The listing builds one solid part. Answer for the finished solid, in the listing's coordinates (mm). Coordinates: 2 decimals unless noted, no trailing zeros. Order: outer loops, then holes, each group sorted by start corner. A loop starts at its lowest first (then second) coordinate and runs counter-clockwise, first axis right, second up. Notation, with made-up numbers: (26.25, -34) -> (39.25, -34) arc R12 cw to (39.25, -12) -> close; hole circle Ø11 at (12.5, 35.25). An arc over 180 degrees is marked (long way). Return JSON: item names as keys, results as strings.
```python
from build123d import *

# Parameters (mm, degrees)
BOSS_EXTRUDE1_DEPTH = 1.25
BOSS_EXTRUDE5_DEPTH = 2.5
SKETCH6_W           = 5
SKETCH6_H           = 4
CUT_EXTRUDE1_DEPTH  = 1.25
CUT_EXTRUDE2_DEPTH  = 2.5


with BuildPart() as part:
    # Sketch2 → Boss-Extrude1 (new body, symmetric)
    with BuildSketch(Plane(origin=(0, 0, 0), x_dir=(1, 0, 0), z_dir=(0, 1, 0))):
        with BuildLine():
            Line((-16.109808132, 35.188266684), (-8.537351427, 63.449059844))
            ThreePointArc((-8.537351427, 63.449059844), (0, 70), (8.537351427, 63.449059844))
            Line((8.537351427, 63.449059844), (16.109808132, 35.188266684))
            ThreePointArc((16.109808132, 35.188266684), (18.609958913, 31.446526618), (22.871288916, 30))
            Line((22.871288916, 30), (37.5, 30))
            ThreePointArc((37.5, 30), (48.106601718, 25.606601718), (52.5, 15))
            Line((52.5, 15), (52.5, -15))
            ThreePointArc((52.5, -15), (40.784271247, -43.284271247), (12.5, -55))
            Line((12.5, -55), (-12.5, -55))
            ThreePointArc((-12.5, -55), (-40.784271247, -43.284271247), (-52.5, -15))
            Line((-52.5, -15), (-52.5, 15))
            ThreePointArc((-52.5, 15), (-48.106601718, 25.606601718), (-37.5, 30))
            Line((-37.5, 30), (-22.871288916, 30))
            ThreePointArc((-22.871288916, 30), (-18.609958913, 31.446526618), (-16.109808132, 35.188266684))
        make_face()
        with BuildLine():
            Line((6.122536861, 62.802012231), (13.694993566, 34.541219072))
            ThreePointArc((13.694993566, 34.541219072), (17.08805534, 29.463143267), (22.871288916, 27.5))
            Line((22.871288916, 27.5), (37.5, 27.5))
            ThreePointArc((37.5, 27.5), (46.338834765, 23.838834765), (50, 15))
            Line((50, 15), (50, -15))
            ThreePointArc((50, -15), (39.016504294, -41.516504294), (12.5, -52.5))
            Line((12.5, -52.5), (-12.5, -52.5))
            ThreePointArc((-12.5, -52.5), (-39.016504294, -41.516504294), (-50, -15))
            Line((-50, -15), (-50, 15))
            ThreePointArc((-50, 15), (-46.338834765, 23.838834765), (-37.5, 27.5))
            Line((-37.5, 27.5), (-22.871288916, 27.5))
            ThreePointArc((-22.871288916, 27.5), (-17.08805534, 29.463143267), (-13.694993566, 34.541219072))
            Line((-13.694993566, 34.541219072), (-6.122536861, 62.802012231))
            ThreePointArc((-6.122536861, 62.802012231), (0, 67.5), (6.122536861, 62.802012231))
        make_face(mode=Mode.SUBTRACT)
    extrude(amount=BOSS_EXTRUDE1_DEPTH, both=True)

    # Sketch5 → Boss-Extrude5 (add)
    with BuildSketch(Plane(origin=(0, 1.25, 0), x_dir=(1, 0, 0), z_dir=(0, 1, 0))):
        with BuildLine():
            ThreePointArc((-50, 15), (-41.161165235, 18.661165235), (-37.5, 27.5))
            ThreePointArc((-37.5, 27.5), (-46.338834765, 23.838834765), (-50, 15))
        make_face()
        with BuildLine():
            ThreePointArc((37.5, 27.5), (41.161165235, 18.661165235), (50, 15))
            ThreePointArc((50, 15), (46.338834765, 23.838834765), (37.5, 27.5))
        make_face()
        with BuildLine():
            ThreePointArc((-50, -15), (-42.291585286, -22.095919329), (-45.973512014, -31.904851181))
            ThreePointArc((-45.973512014, -31.904851181), (-48.979492188, -23.688880811), (-50, -15))
        make_face()
        with BuildLine():
            ThreePointArc((50, -15), (42.291585286, -22.095919329), (45.973512014, -31.904851181))
            ThreePointArc((45.973512014, -31.904851181), (48.979492187, -23.688880811), (50, -15))
        make_face()
    extrude(amount=-BOSS_EXTRUDE5_DEPTH)

    # Sketch6 → Cut-Extrude1 (cut)
    with BuildSketch(Plane(origin=(0, 1.25, 0), x_dir=(1, 0, 0), z_dir=(0, 1, 0))):
        with Locations((0, 68.75)):
            Rectangle(SKETCH6_W, SKETCH6_H)
        with BuildLine():
            Line((-20.493193447, 30.416333701), (-19.643873637, 28.065024308))
            ThreePointArc((-19.643873637, 28.065024308), (-17.08805534, 29.463143267), (-15.076081678, 31.570014354))
            Line((-15.076081678, 31.570014354), (-17.127452004, 32.998957945))
            ThreePointArc((-17.127452004, 32.998957945), (-18.609958913, 31.446526618), (-20.493193447, 30.416333701))
        make_face()
        with BuildLine():
            Line((20.493193447, 30.416333701), (19.643873637, 28.065024308))
            ThreePointArc((19.643873637, 28.065024308), (17.08805534, 29.463143267), (15.076081678, 31.570014354))
            Line((15.076081678, 31.570014354), (17.127452004, 32.998957945))
            ThreePointArc((17.127452004, 32.998957945), (18.609958913, 31.446526618), (20.493193447, 30.416333701))
        make_face()
        with BuildLine():
            Line((-40.784271247, -43.284271247), (-39.016504294, -41.516504294))
            ThreePointArc((-39.016504294, -41.516504294), (-37.189746158, -43.225280064), (-35.253133619, -44.808470449))
            Line((-35.253133619, -44.808470449), (-36.770009194, -46.795701812))
            ThreePointArc((-36.770009194, -46.795701812), (-38.835729235, -45.106965401), (-40.784271247, -43.284271247))
        make_face()
        with BuildLine():
            Line((36.770009194, -46.795701812), (35.253133619, -44.808470449))
            ThreePointArc((35.253133619, -44.808470449), (37.189746158, -43.225280064), (39.016504294, -41.516504294))
            Line((39.016504294, -41.516504294), (40.784271247, -43.284271247))
            ThreePointArc((40.784271247, -43.284271247), (38.835729235, -45.106965401), (36.770009194, -46.795701812))
        make_face()
        with Locations((0, -54)):
            Rectangle(SKETCH6_W, SKETCH6_H)
    extrude(amount=-CUT_EXTRUDE1_DEPTH, mode=Mode.SUBTRACT)

    # Sketch7 → Cut-Extrude2 (cut)
    with BuildSketch(Plane(origin=(0, 1.25, 0), x_dir=(1, 0, 0), z_dir=(0, 1, 0))):
        with BuildLine():
            ThreePointArc((-50, 17.291666667), (-42.781618275, 20.281618275), (-39.791666667, 27.5))
            ThreePointArc((-39.791666667, 27.5), (-46.486148678, 23.986148678), (-50, 17.291666667))
        make_face()
        with BuildLine():
            ThreePointArc((39.791666667, 27.5), (46.486148678, 23.986148678), (50, 17.291666667))
            ThreePointArc((50, 17.291666667), (42.781618275, 20.281618275), (39.791666667, 27.5))
        make_face()
        with BuildLine():
            ThreePointArc((-47.100502093, -29.673283714), (-44.723551432, -22.675178049), (-50, -17.5))
            ThreePointArc((-50, -17.5), (-48.979492187, -23.688880811), (-47.100502093, -29.673283714))
        make_face()
        with BuildLine():
            ThreePointArc((50, -17.5), (48.979492187, -23.688880811), (47.100502093, -29.673283714))
            ThreePointArc((47.100502093, -29.673283714), (44.723551432, -22.675178049), (50, -17.5))
        make_face()
    extrude(amount=-CUT_EXTRUDE2_DEPTH, mode=Mode.SUBTRACT)


solid = part.part
```
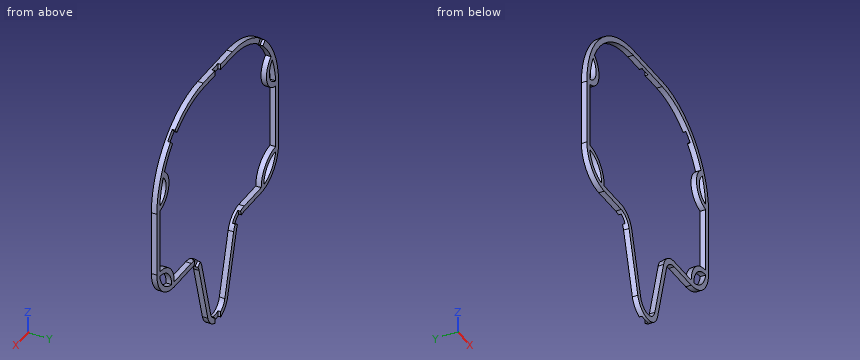
Item 1: The part is cut by section C-C on y = 0.65. Count the separate pieces of the cut face and the enclosed holes in it, plus the area to 3 significant figures.
Answer list:
{"separate pieces": "6", "enclosed holes": "4", "area": "1,040 mm2"}
Item 2: The part is cut by section A-A on x = 1. Determine the outline of the cut face in (y, z).
Answer list:
{"outline": "(-1.25, -69.94) -> (0, -69.94) -> (0, -67.42) -> (-1.25, -67.42) -> close; (-1.25, 52.5) -> (0, 52.5) -> (0, 55) -> (-1.25, 55) -> close"}
Item 3: The part is cut by section D-D on z = 23.5. Determine the outline of the cut face in (x, y).
Answer list:
{"outline": "(-51.59, -1.25) -> (-49.02, -1.25) -> (-49.02, 1.25) -> (-51.59, 1.25) -> close; (-44.58, -1.25) -> (-42.07, -1.25) -> (-42.07, 1.25) -> (-44.58, 1.25) -> close; (42.07, -1.25) -> (44.58, -1.25) -> (44.58, 1.25) -> (42.07, 1.25) -> close; (49.02, -1.25) -> (51.59, -1.25) -> (51.59, 1.25) -> (49.02, 1.25) -> close"}
Item 4: The part is cut by section B-B on z = -12. Determine the outline of the cut face in (x, y).
Answer list:
{"outline": "(-52.5, -1.25) -> (-50, -1.25) -> (-50, 1.25) -> (-52.5, 1.25) -> close; (50, -1.25) -> (52.5, -1.25) -> (52.5, 1.25) -> (50, 1.25) -> close"}
Item 5: Find the intervals of material crossed by probe 1 along X at (y, z) = (-0.5, -11.5); probe 2 along Z at (x, y) = (-43, 0.2); probe 3 along X at (y, z) = (-0.3, 21), in increasing order.
Answer list:
{"probe 1": "-52.5 to -50, 50 to 52.5", "probe 2": "-28.96 to -26.46, -20.07 to -17.14, 20.13 to 28.41, 36.82 to 40.88", "probe 3": "-52.05 to -49.53, -45.36 to -42.62, 42.62 to 45.36, 49.53 to 52.05"}
Item 6: Flat-ended cylindrical pins translate along their axes: pin 1 (0.6 mm diameter, centred on y = 0.5, z = -68, fed in from +X); pin 2 (0.8 mm diameter, centred on x = -30, y = 0.5, fed in from -Z); pin 3 (1.5 mm diameter, centred on x = 18, z = -29.5, fed in from +Y); pin 4 (4 mm diameter, centred on x = -37, z = 45.5, fed in from +Y). Find the tip coordinate at first contact, or state that the pin passes through.
Answer list:
{"pin 1": "x = 5.95", "pin 2": "z = -30", "pin 3": "y = 0", "pin 4": "y = 1.25"}
